Read the model definition and answer for the solid it produces. Units are mm, in the model's axes. A direction names the side the tool comes from. Coordinates: 2 decimals unless noted, no trailing zeros. Loops run counter-clockwise (first coordinate to the right, second up) from the corner with the lowest first, then second, coordinate; pieces in that order, holes last. Notation, with made-up numbers: (59.25, 46) -> (73.25, 46) arc R19 ccw to (73.25, 68) -> close; hole circle Ø8 at (62, -31). An arc over 180 degrees is marked (long way). Answer as a JSON object with one key per item and string values. Group by question number.
1) Flat-ended cylindrical pins translate along their axes: P1, Ø2, axis at y = -15, z = 3.5, coming from the -X side; P2, Ø5, axis at y = 43, z = 4.5, coming from the -X side; P3, Ø3, axis at y = 13, z = 7.5, coming from the +X side. Find the tip coordinate at first contact, or state that the pin passes through.
2) Which of the six approach directions +Z, -Z, +X, -X, +Y, -Y give full straight-line access (tool end or side, diameter ignored) to faces 5 (the face through (-8, 36.695, 5)), 6 (the face through (20.465, -42.449, 4.93)), 7 (the face through (-58.577, 39, 5)), 8 (the face through (47, -47.225, 5)), 9 (the face through (-49.7, 18.86, 4.93))?
3) Section C-C, the plane z = 5.75 is taken. Give the vertices of the cut face in (x, y), plus the area to 3 significant figures.
4) Determine the mould class of faces 1 (the face through (-23.535, -43.058, 4.93)), 2 (the face through (44.18, 45.61, 4.93)), 3 (the face through (57.05, -24.83, 4.93)), 4 (the face through (77.753, -40, 5)) for opening direction Y: released by +Y, released by -Y, zero draft, split by the parting line, or undercut.
5) Section B-B, the plane x = 47 is taken. Give the vertices of the cut face in (y, z), plus the area to 3 significant figures.
6) Consider probe 1 along Y at (x, z) = (-25, 8.75); probe 2 along Y at (x, z) = (-8.5, 2); probe 3 along X at (y, z) = (14, 7.5). Determine where each line is inside the solid, lowest interval first. Write a range as [from, to].
7) Section D-D, the plane y = 31 is taken. Give the vertices of the cut face in (x, z), plus the area to 3 significant figures.
8) Section A-A, the plane y = -41 is taken. Give the vertices of the cut face in (x, z), plus the area to 3 significant figures.
from build123d import *

# Parameters (mm, degrees)
SKETCH1_R           = 18
BOSS_EXTRUDE2_DEPTH = 10


with BuildPart() as part:
    # Sketch1 → Boss-Extrude2 (new body)
    with BuildSketch(Plane.XY):
        Polygon((17.423284477, -47.225403837), (77.753284477, -47.225403837), (77.753284477, -32.225403837), (35.753284477, -17.225403837), (50.753284477, 4.694596163), (50.753284477, 39.694596163), (37.423284477, 51.694596163), (1.423284477, 51.694596163), (1.423284477, 36.694596163), (-18.576715523, 36.694596163), (-18.576715523, 51.694596163), (-58.576715523, 51.694596163), (-58.576715523, 25.694596163), (-40.576715523, 11.834793389), (-40.576715523, -8.165206611), (-58.576715523, -28.165206611), (-70.576715523, -28.165206611), (-70.576715523, -48.165206611), (-20.576715523, -48.165206611), (-26.576715523, -37.805403837), (23.423284477, -37.805403837), align=None)
        with Locations((-8.576715523, 1.334793389)):
            Circle(SKETCH1_R, mode=Mode.SUBTRACT)
    extrude(amount=BOSS_EXTRUDE2_DEPTH)


solid = part.part
Determined:
{
 "1": {"P1": "x = -47.63", "P2": "x = -58.58", "P3": "x = 50.75"},
 "2": {"face 5": "+Z, -Z, +Y", "face 6": "+Z, -Z", "face 7": "+Z, -Z, -X, +Y", "face 8": "+Z, -Z, +X, -Y", "face 9": "+Z, -Z, -X"},
 "3": {"outline": "(-70.58, -48.17) -> (-20.58, -48.17) -> (-26.58, -37.81) -> (23.42, -37.81) -> (17.42, -47.23) -> (77.75, -47.23) -> (77.75, -32.23) -> (35.75, -17.23) -> (50.75, 4.69) -> (50.75, 39.69) -> (37.42, 51.69) -> (1.42, 51.69) -> (1.42, 36.69) -> (-18.58, 36.69) -> (-18.58, 51.69) -> (-58.58, 51.69) -> (-58.58, 25.69) -> (-40.58, 11.83) -> (-40.58, -8.17) -> (-58.58, -28.17) -> (-70.58, -28.17) -> close; hole circle Ø36 at (-8.58, 1.33)", "area": "8,940 mm²"},
 "4": {"face 1": "undercut", "face 2": "released by +Y", "face 3": "undercut", "face 4": "zero draft"},
 "5": {"outline": "(-47.23, 0) -> (-21.24, 0) -> (-21.24, 10) -> (-47.23, 10) -> close; (-0.79, 0) -> (43.07, 0) -> (43.07, 10) -> (-0.79, 10) -> close", "area": "698 mm²"},
 "6": {"probe 1": "[-48.17, -40.53], [-37.81, -6.03], [8.7, 51.69]", "probe 2": "[-37.81, -16.67], [19.33, 36.69]", "probe 3": "[-43.39, -21.37], [4.21, 50.75]"},
 "7": {"outline": "(-58.58, 0) -> (50.75, 0) -> (50.75, 10) -> (-58.58, 10) -> close", "area": "1,090 mm²"},
 "8": {"outline": "(-70.58, 0) -> (-24.73, 0) -> (-24.73, 10) -> (-70.58, 10) -> close; (21.39, 0) -> (77.75, 0) -> (77.75, 10) -> (21.39, 10) -> close", "area": "1,020 mm²"}
}
